Input: part model. Units: mm. Frame: model coordinates. Face numbers are marked on the shaded views. A direction names the side the tool comes from. Give positions to 0.01 mm unless a question says otherwise; leave off trailing zeros. Order: outer loops, then holes, each group sorted by start corner. A loop starts at its lowest first (then second) coordinate and runs counter-clockwise, first axis right, second up. Notation, with made-up numbers: (-20.75, 66) - (19.25, 66) arc R14 cw to (19.25, 90) - close; hole circle Ø7 at (1.5, 89.5). An arc over 180 degrees is marked (long way). Answer in a Markdown table with one row per item. Add a question column.
1. Section query D-D on z = -7. Return loops of the section in (x, y).
2. Section query B-B on x = -3. Return loops of the section in (y, z).
3. Section query C-C on z = 21.5. Return loops of the section in (x, y), and give its area (3 significant figures).
4. Mould query, pull axis Y, two halves, no side actions, for the marked faces 4, 5 and 6. Classes: released by +Y, released by -Y, zero draft, split by the parting line, or undercut.
5. Section query A-A on y = 0. Return loops of the section in (x, z).
6. Access query for the marked faces 1, 2 and 3. Directions: +Z, -Z, +X, -X, +Y, -Y. A direction counts if a zero-diameter tool reaches every point of the face in a straight line with its end or side. Return the directions, or none.
7. Ray query, line 1 (X direction, y = 0, z = 26); line 2 (Y direction, x = -8.5, z = 7.5); line 3 (Y direction, x = 0, z = 38). Return the intervals inside material, ascending. Write a range as [from, to].
8. Contact query for flat-ended pins moving along their axis: pin 1 (2 mm diameter, centred on x = -0.5, z = 31.5, fed in from -Y); pin 2 (13 mm diameter, centred on x = 7.5, y = 1, fed in from -Z); pin 3 (18.5 mm diameter, centred on x = 0, z = -13.35, fed in from -Y); pin 4 (8 mm diameter, centred on x = 6.5, z = 37, fed in from -Y). Output: stop coordinate, or through.
```python
from build123d import *

# Parameters (mm, degrees)
CROQUIS3_W            = 139.658435228
CROQUIS3_H            = 16
CORTAR_EXTRUIR1_DEPTH = 51
CROQUIS4_OUTSIDE_W    = 126.9
CROQUIS4_OUTSIDE_H    = 126.9
CROQUIS4_OUTSIDE_W_2  = 120.050230854
CROQUIS4_OUTSIDE_H_2  = 37.93587295
CORTAR_EXTRUIR2_DEPTH = 107.175895765
CROQUIS5_OUTSIDE_W    = 121.792
CROQUIS5_OUTSIDE_H    = 66.086
CROQUIS5_OUTSIDE_W_2  = 32
CROQUIS5_OUTSIDE_H_2  = 52.876669862
CORTAR_EXTRUIR4_DEPTH = 98.164515307
CROQUIS6_OUTSIDE_W    = 53.342
CROQUIS6_OUTSIDE_H    = 104.342
CROQUIS6_OUTSIDE_R    = 59.713814124
CORTAR_EXTRUIR5_DEPTH = 51
CORTAR_EXTRUIR6_START = -32
CORTAR_EXTRUIR6_DEPTH = 33
CROQUIS8_R            = 8
CORTAR_EXTRUIR7_DEPTH = 65.928309429
CROQUIS9_R            = 8
CORTAR_EXTRUIR8_DEPTH = 51


with BuildPart() as part:
    # Croquis1 → Revolución2 (revolve)
    with BuildSketch(Plane(origin=(0, 0, 0), x_dir=(1, 0, 0), z_dir=(0, 1, 0)), mode=Mode.PRIVATE) as revoluci_n2_sk:
        Polygon((15, -50.205128205), (0, -50.205128205), (0, -18.205128205), (8, -18.205128205), (8, 32.794871795), (46.820512821, 32.794871795), (46.820512821, -27.205128205), (15, -27.205128205), align=None)
    revolve(revoluci_n2_sk.sketch.rotate(Axis((0, 0, -124.102564103), (0, 0, 1)), 180), axis=Axis((0, 0, -124.102564103), (0, 0, 1)))

    # Croquis3 → Cortar-Extruir1 (cut)
    with BuildSketch(Plane(origin=(0, 0, -32.794871795), x_dir=(-1, 0, 0), z_dir=(0, 0, -1))):
        Rectangle(CROQUIS3_W, CROQUIS3_H)
    extrude(amount=-CORTAR_EXTRUIR1_DEPTH, mode=Mode.SUBTRACT)

    # Croquis4 outside → Cortar-Extruir2 (cut, through all)
    with BuildSketch(Plane(origin=(0, 0, -32.794871795), x_dir=(-1, 0, 0), z_dir=(0, 0, -1))):
        Rectangle(CROQUIS4_OUTSIDE_W, CROQUIS4_OUTSIDE_H)
        Rectangle(CROQUIS4_OUTSIDE_W_2, CROQUIS4_OUTSIDE_H_2, mode=Mode.SUBTRACT)
    extrude(amount=-CORTAR_EXTRUIR2_DEPTH, mode=Mode.SUBTRACT)

    # Croquis5 outside → Cortar-Extruir4 (cut, through all)
    with BuildSketch(Plane(origin=(0, 0, -32.794871795), x_dir=(-1, 0, 0), z_dir=(0, 0, -1))):
        Rectangle(CROQUIS5_OUTSIDE_W, CROQUIS5_OUTSIDE_H)
        Rectangle(CROQUIS5_OUTSIDE_W_2, CROQUIS5_OUTSIDE_H_2, mode=Mode.SUBTRACT)
    extrude(amount=-CORTAR_EXTRUIR4_DEPTH, mode=Mode.SUBTRACT)

    # Croquis6 outside → Cortar-Extruir5 (cut)
    with BuildSketch(Plane(origin=(0, 18.967936475, 0), x_dir=(1, 0, 0), z_dir=(0, 1, 0))):
        with Locations((0, -8.705)):
            Rectangle(CROQUIS6_OUTSIDE_W, CROQUIS6_OUTSIDE_H)
        with Locations((0, -27.205128205)):
            Circle(CROQUIS6_OUTSIDE_R, mode=Mode.SUBTRACT)
    extrude(amount=-CORTAR_EXTRUIR5_DEPTH, mode=Mode.SUBTRACT)


with BuildPart() as cortar_extruir5_kept_piece:
    # of the separate pieces the step leaves, the one the design keeps (cortar_extruir5_pieces_kept)
    add(part.part.solids().sort_by_distance((-15, 0, 50.205128205))[0])

    # Cortar-Extruir6: read off the stored shape, not the designer's step
    # Cortar-Extruir6 outline → Cortar-Extruir6 (cut)
    with BuildSketch(Plane(origin=(16, 0, 0), x_dir=(0, 0, -1), z_dir=(1, 0, 0)).offset(CORTAR_EXTRUIR6_START)):
        with BuildLine():
            ThreePointArc((29.810017934, 18.967936475), (31.336160338, 13.54352388), (32.347449433, 8))
            Line((32.347449433, 8), (33.422130035, 0))
            Line((33.422130035, 0), (34, 4.301705749))
            Line((34, 4.301705749), (34, 20))
            Line((34, 20), (29.466668549, 20))
            Line((29.466668549, 20), (29.810017934, 18.967936475))
        make_face()
        with BuildLine():
            Line((34, -4.301705749), (33.422130035, 0))
            Line((33.422130035, 0), (32.347449433, -8))
            ThreePointArc((32.347449433, -8), (31.336160338, -13.54352388), (29.810017934, -18.967936475))
            Line((29.810017934, -18.967936475), (29.466668549, -20))
            Line((29.466668549, -20), (34, -20))
            Line((34, -20), (34, -4.301705749))
        make_face()
    extrude(amount=CORTAR_EXTRUIR6_DEPTH, mode=Mode.SUBTRACT)

    # Croquis8 → Cortar-Extruir7 (cut, through all)
    with BuildSketch(Plane.XZ.offset(18.967936475)):
        with Locations(Location((0, -13.347449433, 0), (0, 0, 270))):
            Circle(CROQUIS8_R)
    extrude(amount=-CORTAR_EXTRUIR7_DEPTH, mode=Mode.SUBTRACT)

    # Croquis9 → Cortar-Extruir8 (cut)
    with BuildSketch(Plane.XY.offset(50.205128205)):
        Circle(CROQUIS9_R)
    extrude(amount=-CORTAR_EXTRUIR8_DEPTH, mode=Mode.SUBTRACT)


solid = cortar_extruir5_kept_piece.part
```
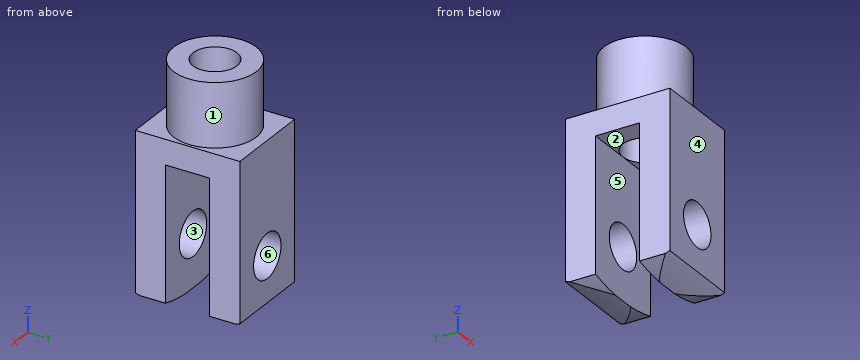
Answer:
| question | item | result |
|---|---|---|
| 1 | outline | (-16, -18.97) - (-4.87, -18.97) - (-4.87, -8) - (-16, -8) - close; (-16, 8) - (-4.87, 8) - (-4.87, 18.97) - (-16, 18.97) - close; (4.87, -18.97) - (16, -18.97) - (16, -8) - (4.87, -8) - close; (4.87, 8) - (16, 8) - (16, 18.97) - (4.87, 18.97) - close |
| 2 | outline | (-18.97, -29.81) arc R60.09 ccw to (-8, -32.35) - (-8, -20.76) - (-18.97, -20.76) - close; (-18.97, -5.93) - (-8, -5.93) - (-8, 18.21) - (-7.42, 18.21) - (-7.42, 50.21) - (-14.7, 50.21) - (-14.7, 27.21) - (-18.97, 27.21) - close; (7.42, 18.21) - (8, 18.21) - (8, -5.93) - (18.97, -5.93) - (18.97, 27.21) - (14.7, 27.21) - (14.7, 50.21) - (7.42, 50.21) - close; (8, -32.35) arc R60.09 ccw to (18.97, -29.81) - (18.97, -20.76) - (8, -20.76) - close |
| 3 | outline | (-16, -18.97) - (16, -18.97) - (16, 18.97) - (-16, 18.97) - close; hole circle Ø16 at (0, 0) |
| 3 | area | 1,010 mm² |
| 4 | face 4 | released by -Y |
| 4 | face 5 | undercut |
| 4 | face 6 | zero draft |
| 5 | outline | (-16, 18.21) - (-8, 18.21) - (-8, 50.21) - (-15, 50.21) - (-15, 27.21) - (-16, 27.21) - close; (8, 18.21) - (16, 18.21) - (16, 27.21) - (15, 27.21) - (15, 50.21) - (8, 50.21) - close |
| 6 | face 1 | +Z |
| 6 | face 2 | -Z, +X, -X |
| 6 | face 3 | +Y, -Y |
| 7 | line 1 | x = [-16, -8], [8, 16] |
| 7 | line 2 | y = [-18.97, -8], [8, 18.97] |
| 7 | line 3 | y = [-15, -8], [8, 15] |
| 8 | pin 1 | stops at y = -15 |
| 8 | pin 2 | stops at z = 18.21 |
| 8 | pin 3 | stops at y = -18.97 |
| 8 | pin 4 | stops at y = -14.79 |
